from build123d import *

# Parameters (mm, degrees)
EXTRUDE_1_DEPTH        = 120
SKETCH_3_W             = 120
SKETCH_3_H             = 20
SM_BASE_FLANGE_1_DEPTH = 3
SM_EDGE_FLANGE_2_DEPTH = 20
EXTRUDE_1_2_DEPTH      = 3


# Sheet-metal steps are written as plain solids
with BuildPart() as part:
    # Sketch 1 → Extrude 1 (new body)
    with BuildSketch(Plane(origin=(0, 0, 0), x_dir=(0, 0, -1), z_dir=(1, 0, 0))):
        Polygon((0, 20), (0, 0), (20, 0), (20, 3), (3, 3), (3, 20), align=None)
    extrude(amount=EXTRUDE_1_DEPTH)



with BuildPart() as body_2:
    # Эскиз3 → Базовая кромка1 (new body)
    with BuildSketch(Plane.XZ):
        with Locations((60, -10)):
            Rectangle(SKETCH_3_W, SKETCH_3_H)
    extrude(amount=-SM_BASE_FLANGE_1_DEPTH)

    # Ребро-кромка2 section (across the edge) → Ребро-кромка2 (add)
    with BuildSketch(Plane(origin=(120.520567051, 0, -20), x_dir=(-0.8191520442889889, -0.5735764363510502, 0), z_dir=(0, 0, 1))):
        with BuildLine():
            Line((-3, 0.520567051), (-3, 23.438298848))
            Line((-3, 23.438298848), (0, 23.438298848))
            Line((0, 23.438298848), (0, 0.520567051))
            ThreePointArc((0, 0.520567051), (0.112989167, 0.058818437), (0.426423564, -0.298584994))
            Line((0.426423564, -0.298584994), (-1.294305745, -2.756041127))
            ThreePointArc((-1.294305745, -2.756041127), (-2.548043333, -1.326427402), (-3, 0.520567051))
        make_face()
    extrude(amount=SM_EDGE_FLANGE_2_DEPTH)


with BuildPart() as part_1:
    add(part.part)

    add(body_2.part)  # Extrude 1 2 merges body 2
    # Эскиз10 → Extrude 1 2 (add)
    with BuildSketch(Plane.XY):
        Polygon((120, 20), (120, 3), (133, 12.102697997), (127.470249606, 20), align=None)
    extrude(amount=-EXTRUDE_1_2_DEPTH)


solid = part_1.part
Source: CAD feature listing. Evaluate the final solid. Frame: model axes, mm. A direction names the side the tool comes from. Round coordinates to 2 decimals unless told otherwise and drop trailing zeros. Write each loop counter-clockwise with the first axis right and the second up, starting at its lowest first coordinate (ties: lowest second). Pieces come first, ordered by that corner, then holes. Notation, with made-up numbers: M 7.5,-6.5 L 57.5,-6.5 A27 cw 57.5,18.5 Z; hole C 79,69 d8. An arc over 180 degrees is marked long. One line per item, written item: value. Start each with the question number.
Item 1: Ray query, L1, parallel to Y at x = 57, z = -15.75; L2, parallel to Z at x = 21, y = 15; L3, parallel to Y at x = 82, z = -1.75. Return the intervals inside material, ascending. Write a range as from..to.
Item 2: Section query B-B (x = 82.5). Return the cut outline in (y, z).
Item 3: Section query D-D (y = 14.5). Return the cut outline in (x, z), plus the area to 3 significant figures.
Item 4: Pin query (flat end, axial travel): pin 1 (8.5 mm diameter, centred on x = 70.5, z = -15, fed in from +Y); pin 2 (5 mm diameter, centred on x = 24, z = -6, fed in from -Y); pin 3 (10 mm diameter, centred on x = 117.5, z = -6, fed in from -Y). Return the tip coordinate at first contact, or that it passes through.
Item 5: Set-up query: faces 4 (the flat face through (75, 1, -20)), 5 (the flat face through (66, 12, -3)), 6 (the flat face through (59, 0, -10)). Return all of +Z, -Z, +X, -X, +Y, -Y with unobstructed straight access to the full face (end or side cutting, diameter ignored); none if empty.
Item 6: Section query C-C (z = -12.5). Return the cut outline in (x, y), plus the area to 3 significant figures.
Item 7: Mould query, pull axis Y, two halves, no side actions, for faces 1 (the flat face through (0, 6.3, -2.5)), 2 (the flat face through (127.48, -9.94, -10.14)), 3 (the flat face through (126.41, 7.49, -1.48)). Classes: pulls with the +Y half, pulls with the -Y half, needs draft (parallel to the pull), parting line crosses it, or undercut.
Item 8: Section query A-A (z = -1.5). Return the cut outline in (x, y), plus the area to 3 significant figures.
Result set:
1. L1: y = 0..3
1. L2: z = -3..0
1. L3: y = 0..20
2. outline: M 0,-20 L 3,-20 L 3,-3 L 20,-3 L 20,0 L 0,0 Z
3. outline: M 0,-3 L 131.32,-3 L 131.32,0 L 0,0 Z
3. area: 394 mm²
4. pin 1: stops at y = 3
4. pin 2: stops at y = 0
4. pin 3: stops at y = -2.83
5. face 4: -Z, +X, -X, +Y, -Y
5. face 5: -Z, +X, -X, +Y
5. face 6: +Z, -Z, -X, -Y
6. outline: M 0,0 L 120,0 A1 cw 120.82,-0.43 L 133.96,-19.2 L 136.42,-17.48 L 123.28,1.29 A4 ccw 120,3 L 0,3 Z
6. area: 436 mm²
7. face 1: needs draft
7. face 2: pulls with the -Y half
7. face 3: undercut
8. outline: M 0,0 L 120,0 A1 cw 120.82,-0.43 L 133.96,-19.2 L 136.42,-17.48 L 123.28,1.29 A4 ccw 120,3 L 133,12.1 L 127.47,20 L 0,20 Z
8. area: 2,620 mm²
